The model under review builds one solid part; all positions refer to its coordinate system, in mm. Give positions to 0.01 mm unless a question says otherwise; leave off trailing zeros. Order: outer loops, then holes, each group sorted by start corner. A loop starts at its lowest first (then second) coordinate and runs counter-clockwise, first axis right, second up. Notation, with made-up numbers: (70, 19) - (80, 19) arc R16 cw to (80, 27) - close; hole circle Ø11 at (46.5, 74.5). An arc over 180 degrees is marked (long way). Put each result on its own line as item: value.
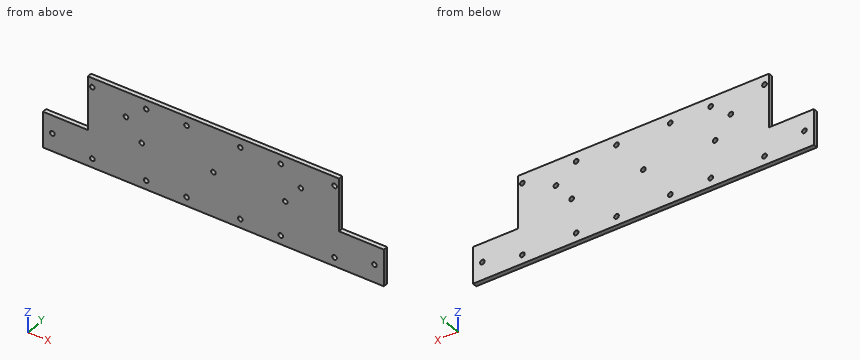
```python
from build123d import *

# Parameters (mm, degrees)
BOSS_EXTRUDE2_DEPTH = 3.175
SKETCH5_R           = 1.651
CUT_EXTRUDE3_DEPTH  = 3.175
SKETCH6_R           = 1.651
CUT_EXTRUDE4_DEPTH  = 3.175
SKETCH7_R           = 1.651
CUT_EXTRUDE5_DEPTH  = 3.81
SKETCH8_R           = 1.651
CUT_EXTRUDE6_DEPTH  = 3.81


with BuildPart() as part:
    # Sketch4 → Boss-Extrude2 (new body)
    with BuildSketch(Plane(origin=(0, 0, 0), x_dir=(1, 0, 0), z_dir=(0, 1, 0))):
        Polygon((-113.15621118, 0), (128.14378882, 0), (128.14378882, -26.103364389), (96.39378882, -26.103364389), (96.39378882, -63.5), (-81.40621118, -63.5), (-81.40621118, -25.4), (-113.15621118, -25.4), align=None)
    extrude(amount=BOSS_EXTRUDE2_DEPTH)

    # Sketch5 → Cut-Extrude3 (cut)
    with BuildSketch(Plane(origin=(0, 3.175, 0), x_dir=(1, 0, 0), z_dir=(0, 1, 0))):
        with Locations(Location((7.49378882, -31.75, 0), (0, 0, 270))):
            Circle(SKETCH5_R)
        with Locations(Location((58.29378882, -31.75, 0), (0, 0, 270))):
            Circle(SKETCH5_R)
        with Locations(Location((-43.30621118, -31.75, 0), (0, 0, 270))):
            Circle(SKETCH5_R)
    extrude(amount=-CUT_EXTRUDE3_DEPTH, mode=Mode.SUBTRACT)

    # Sketch6 → Cut-Extrude4 (cut)
    with BuildSketch(Plane(origin=(0, 3.175, 0), x_dir=(1, 0, 0), z_dir=(0, 1, 0))):
        with Locations(Location((69.40628882, -45.72, 0), (0, 0, 270))):
            Circle(SKETCH6_R)
        with Locations(Location((-54.41871118, -45.72, 0), (0, 0, 270))):
            Circle(SKETCH6_R)
        with Locations(Location((121.47628882, -12.7, 0), (0, 0, 270))):
            Circle(SKETCH6_R)
        with Locations(Location((-106.48871118, -12.7, 0), (0, 0, 270))):
            Circle(SKETCH6_R)
    extrude(amount=-CUT_EXTRUDE4_DEPTH, mode=Mode.SUBTRACT)

    # Sketch7 → Cut-Extrude5 (cut)
    with BuildSketch(Plane(origin=(0, 3.175, 0), x_dir=(1, 0, 0), z_dir=(0, 1, 0))):
        with Locations(Location((93.21878882, -57.0738, 0), (0, 0, 270))):
            Circle(SKETCH7_R)
        with Locations(Location((55.11878882, -57.0738, 0), (0, 0, 270))):
            Circle(SKETCH7_R)
        with Locations(Location((26.54378882, -57.0738, 0), (0, 0, 270))):
            Circle(SKETCH7_R)
        with Locations(Location((-11.55621118, -57.0738, 0), (0, 0, 270))):
            Circle(SKETCH7_R)
        with Locations(Location((-40.13121118, -57.0738, 0), (0, 0, 270))):
            Circle(SKETCH7_R)
        with Locations(Location((-78.23121118, -57.0738, 0), (0, 0, 270))):
            Circle(SKETCH7_R)
    extrude(amount=-CUT_EXTRUDE5_DEPTH, mode=Mode.SUBTRACT)

    # Sketch8 → Cut-Extrude6 (cut)
    with BuildSketch(Plane(origin=(0, 3.175, 0), x_dir=(1, 0, 0), z_dir=(0, 1, 0))):
        with Locations(Location((93.21878882, -6.2738, 0), (0, 0, 270))):
            Circle(SKETCH8_R)
        with Locations(Location((55.11878882, -6.2738, 0), (0, 0, 270))):
            Circle(SKETCH8_R)
        with Locations(Location((26.54378882, -6.2738, 0), (0, 0, 270))):
            Circle(SKETCH8_R)
        with Locations(Location((-11.55621118, -6.2738, 0), (0, 0, 270))):
            Circle(SKETCH8_R)
        with Locations(Location((-40.13121118, -6.2738, 0), (0, 0, 270))):
            Circle(SKETCH8_R)
        with Locations(Location((-78.23121118, -6.2738, 0), (0, 0, 270))):
            Circle(SKETCH8_R)
    extrude(amount=-CUT_EXTRUDE6_DEPTH, mode=Mode.SUBTRACT)


solid = part.part
```
(1) Take a section at C-C, the plane z = 52. Write out the cut boundary in (x, y) (3 decimals), then the cut area to 3 significant figures.
The answers:
outline: (-81.406, 0) - (96.394, 0) - (96.394, 3.175) - (-81.406, 3.175) - close
area: 565 mm^2
(2) Clearance check with flat-ended pins moving along their axes: pin 1 Ø2 at (x, z) = (69.41, 45.72) entering from +Y; pin 2 Ø1 at (y, z) = (2, 46) entering from +X. State where each tip first meets the part, or that it passes through.
The answers:
pin 1: through
pin 2: x = 96.39
(3) Take a section at B-B, the plane x = 103.5. Write out the cut boundary in (y, z) (3 decimals).
The answers:
outline: (0, 0) - (3.175, 0) - (3.175, 26.103) - (0, 26.103) - close
(4) Take a section at A-A, the plane y = 2.2. Count the separate pieces of the cut face and the enclosed holes in it, then the cut area to 3 significant figures.
The answers:
separate pieces: 1
enclosed holes: 19
area: 12,800 mm^2
(5) Wall thickness on L1, parallel to X at y = 0.2, z = 46; L2, parallel to Z at x = -39, y = 2.9; L3, parallel to X at y = 2, z = 41.5: over which ranges is each line inside the solid? List them lowest first.
The answers:
L1: -81.41 to -56.05, -52.79 to 67.78, 71.03 to 96.39
L2: 0 to 5.07, 7.48 to 55.87, 58.28 to 63.5
L3: -81.41 to 96.39
